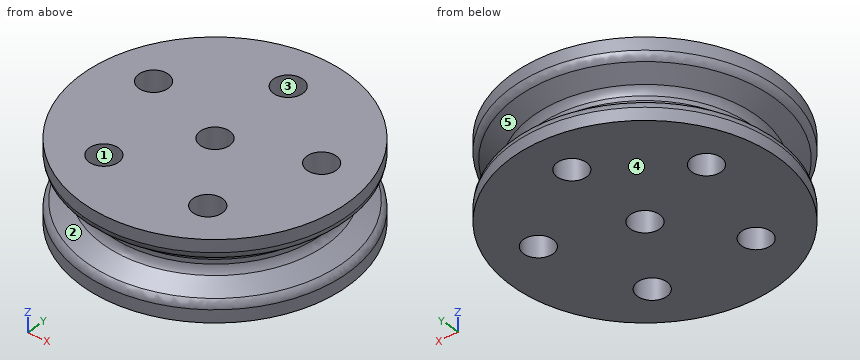
```python
from build123d import *

# Parameters (mm, degrees)
F2_R     = 5
F3_DEPTH = 27
F4_R     = 3


with BuildPart() as f1:
    # F0 (on Right) → F1 (revolve)
    with BuildSketch(Plane.YZ):
        Polygon((-45, -11), (-5, -11), (-5, 16), (-45, 16), (-45, 10), (-36.339746, 5), (-36.339746, 0), (-45, -5), align=None)
    revolve(axis=Axis((0, 0, 0.272177), (0, 0, -1)))

    # F2 (on face) → F3 (cut, through all)
    with BuildSketch(Plane.XY.offset(16)):
        with Locations((0, 30)):
            Circle(F2_R)
        with Locations((-28.531695, 9.27051)):
            Circle(F2_R)
        with Locations((-17.633558, -24.27051)):
            Circle(F2_R)
        with Locations((17.633558, -24.27051)):
            Circle(F2_R)
        with Locations((28.531695, 9.27051)):
            Circle(F2_R)
    extrude(amount=-F3_DEPTH, mode=Mode.SUBTRACT)

    # F4
    f4_edges = [f1.edges().sort_by_distance(p)[0] for p in [
        (0, 36.339746, 0),
        (0, 36.339746, 5),
        (0, 45, -5),
        (0, 45, 10),
    ]]
    fillet(f4_edges, radius=F4_R)


solid = f1.part
```
The listing builds one solid part. Answer for the finished solid, in the listing's coordinates (mm). Face numbers are marked on the shaded views. A direction names the side the tool comes from. Give positions to 0.01 mm unless a question says otherwise; leave off trailing zeros. Order: outer loops, then holes, each group sorted by start corner. A loop starts at its lowest first (then second) coordinate and runs counter-clockwise, first axis right, second up. Notation, with made-up numbers: (7, 0.25) - (15, 0.25) arc R34 cw to (15, 31.25) - close; hole circle Ø6 at (1, -7.75). An arc over 180 degrees is marked (long way). Answer in a Markdown table with one row per item. Add a question column.
Q1. Find the intervals of material crossed by line 1 along Y through (x, z) = (-0.5, 11.75); line 2 along Y through (x, z) = (0, 8); line 3 along X through (y, z) = (10, 10.75), in increasing order. Write a range as [from, to].
Q2. Which of the six approach directions +Z, -Z, +X, -X, +Y, -Y give full straight-line access (tool end or side, diameter ignored) to the marked faces 1 and 2?
Q3. The part is cut by section B-B (z = 7.25). Determine the outline of the cut face in (x, y).
Q4. Given P1, Ø2, axis at y = 21.5, z = 2.5, coming from the -X side; P2, Ø1.5, axis at y = 20, z = -3.5, coming from the +X side; P3, Ø12, axis at y = -35, z = 11, coming from the -X side, each flat-ended and moving along its own axis, determine where each tip first touches the part or whether it passes through.
Q5. For a pull along X with two mould halves and no side action, classify the marked faces 3, 4 and 5 as released by +X, released by -X, zero draft, split by the parting line, or undercut.
Q6. The part is cut by section A-A (x = 0). Give the number of separate pieces and of enclosed holes in the cut face, then the cut area to 3 significant figures.
Q7. The part is cut by section D-D (z = -8.5). Determine the outline of the cut face in (x, y), then the cut area to 3 significant figures.
Determined:
| question | item | result |
|---|---|---|
| 1 | line 1 | y = [-45, -4.97], [4.97, 25.03], [34.97, 45] |
| 1 | line 2 | y = [-41.54, -5], [5, 25], [35, 41.54] |
| 1 | line 3 | x = [-43.71, -33.48], [-23.59, 23.59], [33.48, 43.71] |
| 2 | face 1 | +Z, -Z |
| 2 | face 2 | none |
| 3 | outline | circle Ø80.47 at (0, 0); hole circle Ø10 at (-28.53, 9.27); hole circle Ø10 at (-17.63, -24.27); hole circle Ø10 at (0, 0); hole circle Ø10 at (0, 30); hole circle Ø10 at (17.63, -24.27); hole circle Ø10 at (28.53, 9.27) |
| 4 | P1 | stops at x = -30.01 |
| 4 | P2 | stops at x = 38.89 |
| 4 | P3 | stops at x = -34.38 |
| 5 | face 3 | undercut |
| 5 | face 4 | zero draft |
| 5 | face 5 | split by the parting line |
| 6 | separate pieces | 3 |
| 6 | enclosed holes | 0 |
| 6 | area | 1,720 mm² |
| 7 | outline | circle Ø90 at (0, 0); hole circle Ø10 at (-28.53, 9.27); hole circle Ø10 at (-17.63, -24.27); hole circle Ø10 at (0, 0); hole circle Ø10 at (0, 30); hole circle Ø10 at (17.63, -24.27); hole circle Ø10 at (28.53, 9.27) |
| 7 | area | 5,890 mm² |
